The model under review builds one solid part; all positions refer to its coordinate system, in mm. A direction names the side the tool comes from. Round coordinates to 2 decimals unless told otherwise and drop trailing zeros. Order: outer loops, then holes, each group sorted by start corner. A loop starts at its lowest first (then second) coordinate and runs counter-clockwise, first axis right, second up. Notation, with made-up numbers: (-23, 88.25) -> (-9, 88.25) arc R22 ccw to (-9, 114.25) -> close; hole circle Ø2 at (-37, 34.5). An arc over 180 degrees is marked (long way). Use a Markdown table: item, result. Add a question column.
```python
from build123d import *

# Parameters (mm, degrees)
SKETCH7_R           = 3.5
SKETCH7_R_2         = 1.5
SKETCH7_R_3         = 1
BOSS_EXTRUDE2_DEPTH = 3.5
FILLET1_R           = 10
FILLET2_R           = 1.5


with BuildPart() as part:
    # Sketch7 → Boss-Extrude2 (new body)
    with BuildSketch(Plane.XY):
        with BuildLine():
            Line((3.430427898, 82.694380615), (6, 70))
            Line((6, 70), (44.142135624, 70))
            Line((44.142135624, 70), (93.636038969, 20.506096654))
            Line((93.636038969, 20.506096654), (90.980851591, 17.850909276))
            Line((90.980851591, 17.850909276), (104.533955357, 4.657601188))
            ThreePointArc((104.533955357, 4.657601188), (104.627002282, -4.565177968), (95.403805922, -4.596194078))
            Line((95.403805922, -4.596194078), (81.96877708, 8.838834765))
            Line((81.96877708, 8.838834765), (79.493903346, 6.363961031))
            Line((79.493903346, 6.363961031), (35.857864376, 50))
            Line((35.857864376, 50), (-35.857864376, 50))
            Line((-35.857864376, 50), (-49.445436483, 36.412427894))
            Line((-49.445436483, 36.412427894), (-63.587572106, 50.554563517))
            Line((-63.587572106, 50.554563517), (-44.142135624, 70))
            Line((-44.142135624, 70), (-6, 70))
            Line((-6, 70), (-3.430427898, 82.694380615))
            ThreePointArc((-3.430427898, 82.694380615), (0, 85.5), (3.430427898, 82.694380615))
        make_face()
        with Locations((100, 0)):
            Circle(SKETCH7_R, mode=Mode.SUBTRACT)
        with Locations((0, 82)):
            Circle(SKETCH7_R_2, mode=Mode.SUBTRACT)
        with Locations((0, 60)):
            Circle(SKETCH7_R_2, mode=Mode.SUBTRACT)
        with Locations((86.564971157, 20.506096654)):
            Circle(SKETCH7_R_3, mode=Mode.SUBTRACT)
        with Locations((79.493903346, 13.435028843)):
            Circle(SKETCH7_R_3, mode=Mode.SUBTRACT)
        with Locations((-52.699132326, 47.300867674)):
            Circle(SKETCH7_R_3, mode=Mode.SUBTRACT)
    extrude(amount=BOSS_EXTRUDE2_DEPTH)

    # Fillet1
    fillet1_edges = [part.edges().sort_by_distance(p)[0] for p in [
        (44.142135624, 70, 1.75),
        (35.857864376, 50, 1.75),
        (-35.857864376, 50, 1.75),
        (-44.142135624, 70, 1.75),
    ]]
    fillet(fillet1_edges, radius=FILLET1_R)

    # Fillet2
    fillet2_edges = [part.edges().sort_by_distance(p)[0] for p in [
        (6, 70, 1.75),
        (93.636038969, 20.506096654, 1.75),
        (90.980851591, 17.850909276, 1.75),
        (81.96877708, 8.838834765, 1.75),
        (79.493903346, 6.363961031, 1.75),
        (-49.445436483, 36.412427894, 1.75),
        (-63.587572106, 50.554563517, 1.75),
        (-6, 70, 1.75),
    ]]
    fillet(fillet2_edges, radius=FILLET2_R)


solid = part.part
```
Q1. Wall thickness on line 1 (X direction, y = 47, z = 0.5); line 2 (Y direction, x = 97.5, z = 0.65); line 3 (X direction, y = 39, z = 2.15): over which ranges is each line inside the solid? List them lowest first. Write a range as [from, to].
Q2. Machinability: for faces 5 (the flat face through (23, 70, 2)), 6 (the flat face through (-24, 70, 2)), 7 (the flat face through (0, 50, 2)), which of the approach directions +Z, -Z, +X, -X, +Y, -Y give a long, thin tool a straight path to every point of the face, cutting with its end or side? Answer none if there is none.
Q3. Mouldability with a two-part tool opening along Y and no side actions: class faces 1 (the flat face through (22, 53, 3.5)), 2 (the cylindrical face through (103.233, -1.341, 1.726)), 3 (the cylindrical face through (-43.78, 69.26, 1.77)), 4 (the cylindrical face through (35.49, 49.26, 1.77)) as pulls with the +Y half, pulls with the -Y half, needs draft (parallel to the pull), parting line crosses it, or undercut.
Q4. Add section C-C (x = 55.5). Write out the cut boundary in (y, z).
Q5. Insertion check: pin 1 (1.8 mm diameter, centred on x = -22, z = 2.5, fed in from +Y); pin 2 (1 mm diameter, centred on y = 67, z = 3, fed in from -X); pin 3 (1.8 mm diameter, centred on x = -52.7, y = 47.3, fed in from +Z); pin 4 (2.5 mm diameter, centred on x = 79.49, y = 13.44, fed in from -Z). Each pin has a flat end and moves straight along its axis. Give the tip position at first contact, or say it passes through.
Q6. Add section B-B (x = 100). Write out the cut boundary in (y, z).
Q7. Add section D-D (x = -35). Write out the cut boundary in (y, z).
Q8. Add section A-A (z = 1.4). State how many separate pieces and enclosed holes the cut face has, then the cut area to 3 significant figures.
Report:
| question | item | result |
|---|---|---|
| 1 | line 1 | x = [-60.03, -53.65], [-51.75, -38.86], [38.86, 67.14] |
| 1 | line 2 | y = [-6, -2.45], [2.45, 11.5] |
| 1 | line 3 | x = [-52.03, -46.86], [46.86, 75.14] |
| 2 | face 5 | +Z, -Z, +X, +Y |
| 2 | face 6 | +Z, -Z, -X, +Y |
| 2 | face 7 | +Z, -Z, -Y |
| 3 | face 1 | needs draft |
| 3 | face 2 | undercut |
| 3 | face 3 | pulls with the +Y half |
| 3 | face 4 | pulls with the -Y half |
| 4 | outline | (30.36, 0) -> (58.64, 0) -> (58.64, 3.5) -> (30.36, 3.5) -> close |
| 5 | pin 1 | stops at y = 70 |
| 5 | pin 2 | stops at x = -47.64 |
| 5 | pin 3 | passes through |
| 5 | pin 4 | stops at z = 0 |
| 6 | outline | (-6.5, 0) -> (-3.5, 0) -> (-3.5, 3.5) -> (-6.5, 3.5) -> close; (3.5, 0) -> (9.07, 0) -> (9.07, 3.5) -> (3.5, 3.5) -> close |
| 7 | outline | (49.45, 0) -> (70, 0) -> (70, 3.5) -> (49.45, 3.5) -> close |
| 8 | separate pieces | 1 |
| 8 | enclosed holes | 6 |
| 8 | area | 3,770 mm² |
